from build123d import *

# Parameters (mm, degrees)
SKETCH1_W           = 12.7
SKETCH1_H           = 38.1
SKETCH1_W_2         = 104.775
BOSS_EXTRUDE1_DEPTH = 35.56
SKETCH11_W          = 112.395
SKETCH11_H          = 30.48
CUT_EXTRUDE9_DEPTH  = 35.56
SKETCH5_W           = 12.7
SKETCH5_H           = 5.08
BOSS_EXTRUDE2_DEPTH = 12.7
SKETCH7_W           = 12.7
SKETCH7_H           = 5.08
BOSS_EXTRUDE3_DEPTH = 12.7
SKETCH8_R           = 2.2225
CUT_EXTRUDE6_DEPTH  = 88.497032271
FILLET1_R           = 3.81
SKETCH9_W           = 12.7
SKETCH9_H           = 19.05
CUT_EXTRUDE7_DEPTH  = 90.537814672
SKETCH10_W          = 25.4
SKETCH10_H          = 7.62
CUT_EXTRUDE8_DEPTH  = 8.89


with BuildPart() as part:
    # Sketch1 → Boss-Extrude1 (new body)
    with BuildSketch(Plane(origin=(0, 0, 0), x_dir=(1, 0, 0), z_dir=(0, 1, 0))):
        with Locations((58.7375, 0)):
            Rectangle(SKETCH1_W, SKETCH1_H)
        Rectangle(SKETCH1_W_2, SKETCH1_H)
    extrude(amount=BOSS_EXTRUDE1_DEPTH)

    # Sketch11 → Cut-Extrude9 (cut)
    with BuildSketch(Plane.XY.offset(19.05)):
        with Locations((6.35, 17.78)):
            Rectangle(SKETCH11_W, SKETCH11_H)
    extrude(amount=-CUT_EXTRUDE9_DEPTH, mode=Mode.SUBTRACT)

    # Sketch5 → Boss-Extrude2 (add)
    with BuildSketch(Plane.XZ):
        with Locations((-30.1625, 16.51)):
            Rectangle(SKETCH5_W, SKETCH5_H)
        with Locations((33.3375, 16.51)):
            Rectangle(SKETCH5_W, SKETCH5_H)
    extrude(amount=BOSS_EXTRUDE2_DEPTH)

    # Sketch7 → Boss-Extrude3 (add)
    with BuildSketch(Plane(origin=(0, 35.56, 0), x_dir=(1, 0, 0), z_dir=(0, 1, 0))):
        with Locations((-17.4625, -16.51)):
            Rectangle(SKETCH7_W, SKETCH7_H)
    extrude(amount=BOSS_EXTRUDE3_DEPTH)

    # Sketch8 → Cut-Extrude6 (cut, through all)
    with BuildSketch(Plane(origin=(0, 0, 13.97), x_dir=(-1, 0, 0), z_dir=(0, 0, -1))):
        with Locations((-33.3375, -6.35)):
            Circle(SKETCH8_R)
        with Locations((30.1625, -6.35)):
            Circle(SKETCH8_R)
        with Locations((17.4625, 41.91)):
            Circle(SKETCH8_R)
    extrude(amount=-CUT_EXTRUDE6_DEPTH, mode=Mode.SUBTRACT)

    # Fillet1
    fillet1_edges = [part.edges().sort_by_distance(p)[0] for p in [
        (65.0875, 35.56, 0),
        (62.5475, 2.54, 1.27),
        (62.5475, 33.02, 1.27),
        (-49.8475, 33.02, 1.27),
        (-49.8475, 2.54, 1.27),
        (-52.3875, 35.56, 0),
        (-36.5125, 0, 16.51),
        (-23.8125, -12.7, 16.51),
        (-36.5125, -12.7, 16.51),
        (-23.8125, 0, 16.51),
        (39.6875, 0, 16.51),
        (26.9875, 0, 16.51),
        (39.6875, -12.7, 16.51),
        (26.9875, -12.7, 16.51),
        (-11.1125, 35.56, 16.51),
        (-23.8125, 35.56, 16.51),
        (-52.3875, 0, 0),
        (-11.1125, 48.26, 16.51),
        (-23.8125, 48.26, 16.51),
        (65.0875, 0, 0),
    ]]
    fillet(fillet1_edges, radius=FILLET1_R)

    # Sketch9 → Cut-Extrude7 (cut, through all)
    with BuildSketch(Plane(origin=(0, 0, -19.05), x_dir=(-1, 0, 0), z_dir=(0, 0, -1))):
        with Locations((-58.7375, 17.78)):
            Rectangle(SKETCH9_W, SKETCH9_H)
    extrude(amount=-CUT_EXTRUDE7_DEPTH, mode=Mode.SUBTRACT)

    # Sketch10 → Cut-Extrude8 (cut)
    with BuildSketch(Plane(origin=(0, 35.56, 0), x_dir=(1, 0, 0), z_dir=(0, 1, 0))):
        Polygon((-7.3025, -19.05), (3.712545586, -19.05), (3.712545586, -11.43), (-8.987454414, -11.43), (-8.987454414, -13.97), (-7.3025, -13.97), align=None)
        with Locations((16.412545586, -15.24)):
            Rectangle(SKETCH10_W, SKETCH10_H)
    extrude(amount=-CUT_EXTRUDE8_DEPTH, mode=Mode.SUBTRACT)


solid = part.part
CAD build for the part. Positions are in the model's coordinates, mm. A direction names the side the tool comes from. Coordinates: 2 decimals unless noted, no trailing zeros. Write each loop counter-clockwise with the first axis right and the second up, starting at its lowest first coordinate (ties: lowest second). Pieces come first, ordered by that corner, then holes. Notation, with made-up numbers: M 42,-9 L 73,-9 A16 ccw 73,2 Z; hole C 12.25,66 d3. An arc over 180 degrees is marked long. Return JSON: item names as keys, results as strings.
Item 1: Slice it at C-C, the plane x = 34. Write the cut outline in (y, z).
Findings below:
{"outline": "M -12.7,13.97 L -8.47,13.97 L -8.47,19.05 L -12.7,19.05 Z; M -4.23,13.97 L 0,13.97 L 0,-19.05 L 35.56,-19.05 L 35.56,19.05 L 33.02,19.05 L 33.02,-16.51 L 2.54,-16.51 L 2.54,19.05 L -4.23,19.05 Z"}
Item 2: Which spindle directions (+Z, -Z, +X, -X, +Y, -Y) get a long thin tool onto all of the face, cutting with end or side? Do faces 1 (the flat face through (6, 2.54, 2)), 2 (the flat face through (-8.987, 34, 13)), 3 (the flat face through (63, 8.255, -4)), 4 (the cylindrical face through (-22.73, 47.11, 16.47)), 5 (the cylindrical face through (-22.67, -1.09, 16.55)). Say none if no direction does.
Findings below:
{"face 1": "+Z", "face 2": "+Y", "face 3": "+Z, -Z, +X", "face 4": "+Z, -Z, -X, +Y", "face 5": "+Z, -Z, -Y"}
Item 3: Drop flat-ended pins along their axis: pin 1 Ø4 at (x, y) = (33, -4.5) entering from -Z; pin 2 Ø5 at (x, y) = (-30.5, 8.5) entering from +Z; pin 3 Ø19 at (x, z) = (20.5, -4.5) entering from +Y. Give the stop position or say it passes through.
Findings below:
{"pin 1": "stops at z = 13.97", "pin 2": "stops at z = -16.51", "pin 3": "stops at y = 35.56"}
Item 4: Probe line 1 (X direction, y = -6, z = 15); line 2 (Y direction, x = 47.5, z = 5.5); line 3 (X direction, y = 3.5, z = -3.5). List the from-to ranges inside material, lowest first. Write a range as from..to.
Findings below:
{"line 1": "x = -36.51..-32.36, -27.97..-23.81, 26.99..31.14, 35.53..39.69", "line 2": "y = 0..2.54, 33.02..35.56", "line 3": "x = -52.37..-48.57, 61.27..65.07"}
Item 5: Slice it at D-D, the plane x = -44.5. Write the cut outline in (y, z), and give its area (3 significant figures).
Findings below:
{"outline": "M 0,-19.05 L 35.56,-19.05 L 35.56,19.05 L 33.02,19.05 L 33.02,-16.51 L 2.54,-16.51 L 2.54,19.05 L 0,19.05 Z", "area": "271 mm2"}
Item 6: Slice it at A-A, the plane y = -6.35. State how many separate pieces and enclosed holes the cut face has, and give its area (3 significant figures).
Findings below:
{"separate pieces": "4", "enclosed holes": "0", "area": "83.9 mm2"}
Item 7: Two-plate mould, pull along X, no slides. Class faces 6 (the cylindrical face through (-51.242, 34.474, -0.267)), 7 (the cylindrical face through (40.83, -1.09, 16.55)), 8 (the cylindrical face through (-24.958, -11.614, 16.546)): +X half, -X half, draft (parallel to the pull), parting line (faces both ways), or undercut.
Findings below:
{"face 6": "-X half", "face 7": "+X half", "face 8": "undercut"}
